Autodesk Inventor part; units mm, degrees
ref_plane "YZ Plane" through (0, 0, 0) normal (1, 0, 0) x (0, 1, 0)
ref_plane "XZ Plane" through (0, 0, 0) normal (0, 1, 0) x (-1, 0, 0)
ref_plane "XY Plane" through (0, 0, 0) normal (0, 0, 1) x (1, 0, 0)
sketch "Sketch1" plane through (0, 0, 0) normal (1, 0, 0) x (0, 1, 0)
  line L0 (-13, 24) -> (-13, -24)
  line L1 (-13, -24) -> (13, -24)
  line L2 (13, -24) -> (13, 24)
  line L3 (13, 24) -> (-13, 24)
  line L4 (-13, 24) -> (13, -24) construction
  line L5 (-13, -24) -> (13, 24) construction
  point P0 (0, 0)
  dimension "d0" = 48
  dimension "d1" = 26
extrude "Extrusion1" add sketch "Sketch1" along normal blind 5
sketch "Sketch2" plane through (5, 0, 0) normal (1, 0, 0) x (0, 0, -1)
  circle A0 centre (17.4055, -5) radius 1.5
  line L0 (3.065, 0) -> (34.1813, 0)
  circle A1 centre (17.4055, 5) radius 1.5
  point P0 (0, 0)
  dimension "d5" = 3
  dimension "d11" = 17.4055
  dimension "d12" = 5
extrude "Extrusion2" cut sketch "Sketch2" against normal blind 5 contours A0
thread "Thread1"
mirror "Mirror1" about plane through (0, 0, 0) normal (0, 0, 1) of "Extrusion2"
fillet "Fillet1" radius 0.6 12 edges at (5, -13, 0) (0, -13, 0) (2.5, -13, -24) (5, 0, -24) (0, 0, -24) (2.5, 13, -24) (5, 13, 0) (0, 13, 0) (2.5, 13, 24) (5, 0, 24) (2.5, -13, 24) (0, 0, 24)
mirror "Mirror2" about plane through (0, 0, 0) normal (0, 1, 0) of "Extrusion2", "Mirror1"
properties part number "Clamp Plate V2"
The listing builds one solid part. Answer for the finished solid, in the listing's coordinates (mm). Coordinates: 2 decimals unless noted, no trailing zeros. Loops run counter-clockwise (first coordinate to the right, second up) from the corner with the lowest first, then second, coordinate; pieces in that order, holes last.
1) Find section C-C on x = 3.05. Write down the section's boundary in (y, z).
2) Determine the mould class of faces 1 (the face through (2, -13, 0)), 2 (the face through (2.535, -5.451, 18.836)), 3 (the face through (2.535, 4.549, 18.836)), 4 (the face through (2, 0, -24)) for opening direction Z: pulls with the +Z half, pulls with the -Z half, needs draft (parallel to the pull), parting line crosses it, or undercut.
3) Find the intervals of material crossed by L1, parallel to Z at x = 2.35, y = 5; L2, parallel to Y at x = 2, z = 18; L3, parallel to Z at x = 3.8, y = -4, in increasing order.
4) Find section A-A on z = -17.5. Write down the section's boundary in (x, y).
5) Find section B-B on y = -5. Write down the section's boundary in (x, z).
6) Flat-ended cylindrical pins translate along their axes: pin 1 Ø2.5 at (y, z) = (5, 17.41) entering from +X; pin 2 Ø6 at (y, z) = (-0.5, -11.5) entering from -X. Find the tip coordinate at first contact, or state that the pin passes through.
Values:
1. outline: (-13, -23.4) arc R0.6 ccw to (-12.4, -24) - (12.4, -24) arc R0.6 ccw to (13, -23.4) - (13, 23.4) arc R0.6 ccw to (12.4, 24) - (-12.4, 24) arc R0.6 ccw to (-13, 23.4) - close; hole circle Ø3 at (-5, -17.41); hole circle Ø3 at (-5, 17.41); hole circle Ø3 at (5, -17.41); hole circle Ø3 at (5, 17.41)
2. face 1: needs draft
2. face 2: undercut
2. face 3: undercut
2. face 4: pulls with the -Z half
3. L1: z = -24 to -18.91, -15.91 to 15.91, 18.91 to 24
3. L2: y = -13 to -6.38, -3.62 to 3.62, 6.38 to 13
3. L3: z = -24 to -18.52, -16.29 to 16.29, 18.52 to 24
4. outline: (0, -12.4) arc R0.6 ccw to (0.6, -13) - (4.4, -13) arc R0.6 ccw to (5, -12.4) - (5, -6.5) - (0, -6.5) - close; (0, -3.5) - (5, -3.5) - (5, 3.5) - (0, 3.5) - close; (0, 6.5) - (5, 6.5) - (5, 12.4) arc R0.6 ccw to (4.4, 13) - (0.6, 13) arc R0.6 ccw to (0, 12.4) - close
5. outline: (0, -23.4) arc R0.6 ccw to (0.6, -24) - (4.4, -24) arc R0.6 ccw to (5, -23.4) - (5, -18.91) - (0, -18.91) - close; (0, -15.91) - (5, -15.91) - (5, 15.91) - (0, 15.91) - close; (0, 18.91) - (5, 18.91) - (5, 23.4) arc R0.6 ccw to (4.4, 24) - (0.6, 24) arc R0.6 ccw to (0, 23.4) - close
6. pin 1: passes through
6. pin 2: stops at x = 0
